The drawing under review shows one solid part. Ordinate dimensions are in mm from its lowest x, y, z. Round coordinates to 2 decimals unless told otherwise and drop trailing zeros. Write each loop counter-clockwise with the first axis right and the second up, starting at its lowest first coordinate (ties: lowest second). Pieces come first, ordered by that corner, then holes.
Item 1: Add section A-A (x = 20). Give the boundary of the cut face in (y, z).
Item 2: To check wall thickness, follow L1, parallel to Z at x = 20, y = 1.15; L2, parallel to Z at x = 19, y = 0.9; L3, parallel to X at y = 2.35, z = 21 (1 decimal). State the ranges of each line that lie inside material, in increasing order.
Item 3: Clearance check with a flat-ended pin moving along its axis: pin 1 Ø6 at (x, z) = (20, 19.97) entering from +Y. State where the tip first meets the part, or that it passes through.
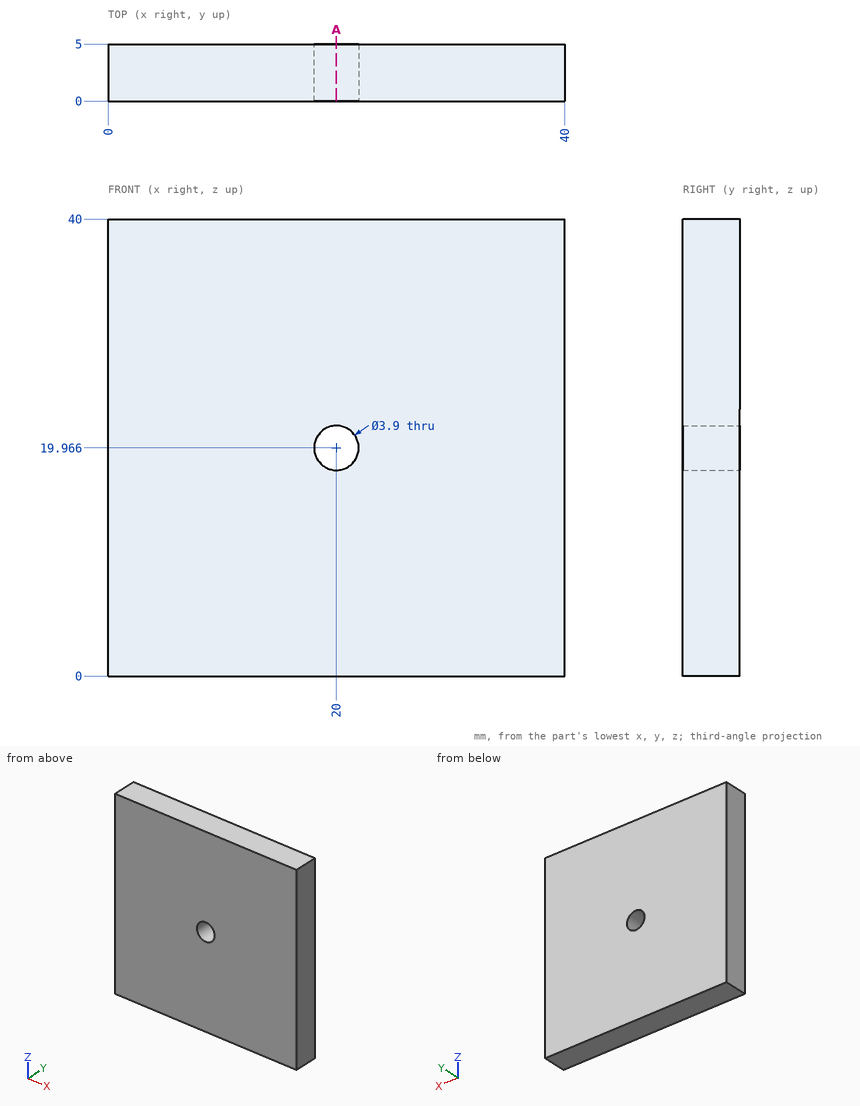
Numbers:
1. outline: (0, 0) - (5, 0) - (5, 18.02) - (0, 18.02) - close; (0, 21.92) - (5, 21.92) - (5, 40) - (0, 40) - close
2. L1: z = 0 to 18.02, 21.92 to 40
2. L2: z = 0 to 18.29, 21.64 to 40
2. L3: x = 0 to 18.3, 21.7 to 40
3. pin 1: stops at y = 5
